Here's how the part is built. I have some questions about the finished solid (model axes, mm). Face numbers are marked on the shaded views. A direction names the side the tool comes from. Round coordinates to 2 decimals unless told otherwise and drop trailing zeros. Order: outer loops, then holes, each group sorted by start corner. A loop starts at its lowest first (then second) coordinate and runs counter-clockwise, first axis right, second up. Notation, with made-up numbers: (40, 29) -> (57, 29) arc R34 ccw to (57, 65) -> close; hole circle Ø5 at (59.25, 11.5). An arc over 180 degrees is marked (long way). Use a Markdown table: item, result. Add a question column.
(1) Thinking about a two-plate mould opening in Z: for the marked faces 6, 7, 8 and 9, which applies, pulls with the +Z half, pulls with the -Z half, needs draft (parallel to the pull), parting line crosses it, or undercut?
(2) I want a section at B-B, the plane x = -63. Please give me the cut outline in (y, z).
(3) If I drill on probe 1 along Z at (x, y) = (83.5, 28.5); probe 2 along Z at (x, y) = (-116, 19); probe 3 along X at (y, z) = (33, -67), over which ranges is the centre line in solid material (lowest first)?
(4) On a 3-axis mill with a long thin cutter (end or side, diameter ignored), from which of +Z, -Z, +X, -X, +Y, -Y can I reach the whole of each face in a straight line? I mean the marked faces 1, 2, 3, 4 and 5. Say none if no direction works.
(5) I'm going to push flat-ended pins straight in: P1, Ø4, axis at x = -28, z = 94.5, coming from the +Y side; P2, Ø1.5, axis at y = 21.5, z = 66, coming from the -X side; P3, Ø8, axis at y = 7, z = 74, coming from the -X side. Where does each tip first touch, or does it pass through?
(6) I want a section at C-C, the plane x = -129.26. Give the number of separate pieces and of enclosed holes in the cut face, then the cut area to 3 significant figures.
(7) I want a section at A-A, the plane z = 35.5. Please give me the cut outline in (x, y).
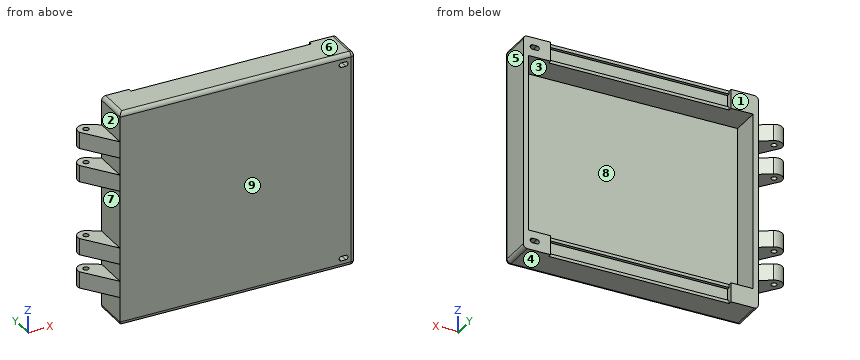
from build123d import *

# Parameters (mm, degrees)
SKETCH1_W               = 228.04
SKETCH1_H               = 209.32
BOSS_EXTRUDE1_DEPTH     = 33.5
SKETCH2_W               = 218.04
SKETCH2_H               = 171.92
CUT_EXTRUDE1_DEPTH      = 28.5
SKETCH4_W               = 175
SKETCH4_H               = 18.7
CUT_EXTRUDE2_DEPTH      = 3.35
SKETCH5_W               = 175
SKETCH5_H               = 12.7
CUT_EXTRUDE3_DEPTH      = 3
SKETCH6_W               = 175
SKETCH6_H               = 18.7
CUT_EXTRUDE4_DEPTH      = 3.35
SKETCH7_W               = 175
SKETCH7_H               = 12.7
CUT_EXTRUDE5_DEPTH      = 3
SKETCH9_R               = 2.75
BOSS_EXTRUDE2_DEPTH     = 8
MIRROR2_COPY_1_SKETCH_R = 2.75
MIRROR2_COPY_1_DEPTH    = 8
CUT_EXTRUDE6_DEPTH      = 33.5
FILLET3_R               = 3.81


with BuildPart() as part:
    # Sketch1 → Boss-Extrude1 (new body)
    with BuildSketch(Plane(origin=(0, 0, 0), x_dir=(1, 0, 0), z_dir=(0, 1, 0))):
        Rectangle(SKETCH1_W, SKETCH1_H)
    extrude(amount=BOSS_EXTRUDE1_DEPTH)

    # Sketch2 → Cut-Extrude1 (cut)
    with BuildSketch(Plane(origin=(0, 33.5, 0), x_dir=(1, 0, 0), z_dir=(0, 1, 0))):
        Rectangle(SKETCH2_W, SKETCH2_H)
    extrude(amount=-CUT_EXTRUDE1_DEPTH, mode=Mode.SUBTRACT)

    # Sketch4 → Cut-Extrude2 (cut)
    with BuildSketch(Plane(origin=(0, 33.5, 0), x_dir=(1, 0, 0), z_dir=(0, 1, 0))):
        with Locations((0, -95.31)):
            Rectangle(SKETCH4_W, SKETCH4_H)
    extrude(amount=-CUT_EXTRUDE2_DEPTH, mode=Mode.SUBTRACT)

    # Sketch5 → Cut-Extrude3 (cut)
    with BuildSketch(Plane(origin=(0, 30.15, 0), x_dir=(1, 0, 0), z_dir=(0, 1, 0))):
        with Locations((0, -95.31)):
            Rectangle(SKETCH5_W, SKETCH5_H)
    extrude(amount=-CUT_EXTRUDE3_DEPTH, mode=Mode.SUBTRACT)

    # Sketch6 → Cut-Extrude4 (cut)
    with BuildSketch(Plane(origin=(0, 33.5, 0), x_dir=(1, 0, 0), z_dir=(0, 1, 0))):
        with Locations((0, 95.31)):
            Rectangle(SKETCH6_W, SKETCH6_H)
    extrude(amount=-CUT_EXTRUDE4_DEPTH, mode=Mode.SUBTRACT)

    # Sketch7 → Cut-Extrude5 (cut)
    with BuildSketch(Plane(origin=(0, 30.15, 0), x_dir=(1, 0, 0), z_dir=(0, 1, 0))):
        with Locations((0, 95.31)):
            Rectangle(SKETCH7_W, SKETCH7_H)
    extrude(amount=-CUT_EXTRUDE5_DEPTH, mode=Mode.SUBTRACT)

    # Sketch9 → Boss-Extrude2 (add, symmetric)
    with BuildSketch(Plane.XY.offset(-35.96)):
        with BuildLine():
            Line((-114.02, 0), (-136.905438379, 30.980124606))
            ThreePointArc((-136.905438379, 30.980124606), (-134.276086797, 39.796139551), (-125.095451514, 40.389051887))
            Line((-125.095451514, 40.389051887), (-114.02, 33.5))
            Line((-114.02, 33.5), (-114.02, 0))
        make_face()
        with Locations((-129.26, 33.5)):
            Circle(SKETCH9_R, mode=Mode.SUBTRACT)
    boss_extrude2 = extrude(amount=BOSS_EXTRUDE2_DEPTH, both=True)

    # Mirror1: Boss-Extrude2 across plane
    add(boss_extrude2.mirror(Plane.XY.offset(-52.33)))

    # Mirror2: Boss-Extrude2 across plane
    add(boss_extrude2.mirror(Plane.XY))

    # Mirror2 copy 1 sketch → Mirror2 copy 1 (add, symmetric)
    with BuildSketch(Plane.XY.offset(68.7)):
        with BuildLine():
            Line((-114.02, 0), (-136.905438379, 30.980124606))
            ThreePointArc((-136.905438379, 30.980124606), (-134.276086797, 39.796139551), (-125.095451514, 40.389051887))
            Line((-125.095451514, 40.389051887), (-114.02, 33.5))
            Line((-114.02, 33.5), (-114.02, 0))
        make_face()
        with Locations((-129.26, 33.5)):
            Circle(MIRROR2_COPY_1_SKETCH_R, mode=Mode.SUBTRACT)
    extrude(amount=MIRROR2_COPY_1_DEPTH, both=True)

    # Sketch11 → Cut-Extrude6 (cut)
    with BuildSketch(Plane(origin=(0, 33.5, 0), x_dir=(1, 0, 0), z_dir=(0, 1, 0))):
        with BuildLine():
            Line((100.76, 93.11), (105.160002263, 93.11))
            ThreePointArc((105.160002263, 93.11), (107.360001132, 95.310001132), (105.16, 97.51))
            Line((105.16, 97.51), (100.76, 97.51))
            ThreePointArc((100.76, 97.51), (98.56, 95.31), (100.76, 93.11))
        make_face()
    cut_extrude6 = extrude(amount=-CUT_EXTRUDE6_DEPTH, mode=Mode.SUBTRACT)

    # Mirror3: Cut-Extrude6 across plane
    add(cut_extrude6.mirror(Plane.XY), mode=Mode.SUBTRACT)

    # Fillet3
    fillet3_edges = [part.edges().sort_by_distance(p)[0] for p in [
        (0, 0, 104.66),
        (0, 0, -104.66),
        (114.02, 0, 0),
        (114.02, 16.75, 104.66),
        (-114.02, 16.75, 104.66),
        (-114.02, 16.75, -104.66),
        (114.02, 16.75, -104.66),
    ]]
    fillet(fillet3_edges, radius=FILLET3_R)


solid = part.part
Taken from the geometry:
| question | item | result |
|---|---|---|
| 1 | face 6 | pulls with the +Z half |
| 1 | face 7 | undercut |
| 1 | face 8 | undercut |
| 1 | face 9 | needs draft |
| 2 | outline | (0, -100.85) arc R3.81 ccw to (3.81, -104.66) -> (30.15, -104.66) -> (30.15, -101.66) -> (27.15, -101.66) -> (27.15, -88.96) -> (30.15, -88.96) -> (30.15, -85.96) -> (5, -85.96) -> (5, 85.96) -> (30.15, 85.96) -> (30.15, 88.96) -> (27.15, 88.96) -> (27.15, 101.66) -> (30.15, 101.66) -> (30.15, 104.66) -> (3.81, 104.66) arc R3.81 ccw to (0, 100.85) -> close |
| 3 | probe 1 | z = -104.66 to -101.66, -88.96 to -85.96, 85.96 to 88.96, 101.66 to 104.66 |
| 3 | probe 2 | z = -76.7 to -60.7, -43.96 to -27.96, 27.96 to 43.96, 60.7 to 76.7 |
| 3 | probe 3 | x = -137.29 to -131.96, -126.56 to -109.02, 109.02 to 114.02 |
| 4 | face 1 | +Z, -Z, +X, +Y |
| 4 | face 2 | +Z, -X, +Y, -Y |
| 4 | face 3 | +Y |
| 4 | face 4 | -Z, +X, -X, +Y, -Y |
| 4 | face 5 | +Z, -Z, +X, +Y, -Y |
| 5 | P1 | stops at y = 27.15 |
| 5 | P2 | stops at x = -130.46 |
| 5 | P3 | stops at x = -122.15 |
| 6 | separate pieces | 8 |
| 6 | enclosed holes | 0 |
| 6 | area | 987 mm2 |
| 7 | outline | (-136.91, 30.98) -> (-114.02, 0) -> (110.21, 0) arc R3.81 ccw to (114.02, 3.81) -> (114.02, 33.5) -> (109.02, 33.5) -> (109.02, 5) -> (-109.02, 5) -> (-109.02, 33.5) -> (-114.02, 33.5) -> (-125.1, 40.39) arc R8.05 ccw to start; hole circle Ø5.5 at (-129.26, 33.5) |
